Read the model definition and answer for the solid it produces. Units are mm, in the model's axes. A direction names the side the tool comes from. Coordinates: 2 decimals unless noted, no trailing zeros. Loops run counter-clockwise (first coordinate to the right, second up) from the corner with the lowest first, then second, coordinate; pieces in that order, holes last. Notation, with made-up numbers: (-25.75, 38) -> (0.25, 38) arc R17 cw to (0.25, 66) -> close; hole circle Ø1 at (41.25, -32). An arc over 180 degrees is marked (long way). Answer in a Markdown table with one row per item.
```python
from build123d import *

# Parameters (mm, degrees)
SKETCH1_W           = 109.5
SKETCH1_H           = 60.5
BOSS_EXTRUDE1_DEPTH = 14
SKETCH2_W           = 103.5
SKETCH2_H           = 54.5
CUT_EXTRUDE1_DEPTH  = 12
SKETCH4_W           = 13
SKETCH4_H           = 9
SKETCH4_W_2         = 10.2
CUT_EXTRUDE2_DEPTH  = 115.460964962
SKETCH5_W           = 4.5
SKETCH5_H           = 100
BOSS_EXTRUDE3_DEPTH = 4.8
BOSS_EXTRUDE7_DEPTH = 14
SKETCH9_W           = 50
SKETCH9_H           = 37.5
BOSS_EXTRUDE8_DEPTH = 4


with BuildPart() as part:
    # Sketch1 → Boss-Extrude1 (new body)
    with BuildSketch(Plane(origin=(0, 0, 0), x_dir=(1, 0, 0), z_dir=(0, 1, 0))):
        Rectangle(SKETCH1_W, SKETCH1_H)
    extrude(amount=BOSS_EXTRUDE1_DEPTH)

    # Sketch2 → Cut-Extrude1 (cut)
    with BuildSketch(Plane(origin=(0, 14, 0), x_dir=(1, 0, 0), z_dir=(0, 1, 0))):
        Rectangle(SKETCH2_W, SKETCH2_H)
    extrude(amount=-CUT_EXTRUDE1_DEPTH, mode=Mode.SUBTRACT)

    # Sketch4 → Cut-Extrude2 (cut, through all)
    with BuildSketch(Plane(origin=(54.75, 0, 0), x_dir=(0, 0, -1), z_dir=(1, 0, 0))):
        with Locations((-11.55, 9.5)):
            Rectangle(SKETCH4_W, SKETCH4_H)
        with Locations((18.25, 9.5)):
            Rectangle(SKETCH4_W_2, SKETCH4_H)
    extrude(amount=-CUT_EXTRUDE2_DEPTH, mode=Mode.SUBTRACT)

    # Sketch5 → Boss-Extrude3 (add)
    with BuildSketch(Plane.XZ):
        with Locations((-6.65, 19.75)):
            Rectangle(SKETCH5_W, SKETCH5_H)
    boss_extrude3 = extrude(amount=BOSS_EXTRUDE3_DEPTH)

    # Mirror1: Boss-Extrude3 across plane
    add(boss_extrude3.mirror(Plane(origin=(0, 0, 0), x_dir=(0, 0, 1), z_dir=(1, 0, 0))))

    # Sketch6 → Boss-Extrude7 (add)
    with BuildSketch(Plane(origin=(0, 0, 0), x_dir=(1, 0, 0), z_dir=(0, 1, 0))):
        Polygon((-0.75, -30.25), (-0.75, -69.75), (-54.75, -69.75), (-54.75, -30.25), (-52.75, -30.25), (-52.75, -67.75), (-2.75, -67.75), (-2.75, -30.25), align=None)
        Polygon((54.75, -30.25), (54.75, -69.75), (0.75, -69.75), (0.75, -30.25), (2.75, -30.25), (2.75, -67.75), (52.75, -67.75), (52.75, -30.25), align=None)
    extrude(amount=BOSS_EXTRUDE7_DEPTH)

    # Sketch9 → Boss-Extrude8 (add)
    with BuildSketch(Plane(origin=(0, 0, 0), x_dir=(1, 0, 0), z_dir=(0, 1, 0))):
        with Locations((-27.75, -49)):
            Rectangle(SKETCH9_W, SKETCH9_H)
        with Locations((27.75, -49)):
            Rectangle(SKETCH9_W, SKETCH9_H)
    extrude(amount=BOSS_EXTRUDE8_DEPTH)


solid = part.part
```
1. A cutting plane is placed at A-A on y = -3.25. Give the vertices of the cut face in (x, z).
A:
| item | result |
|---|---|
| outline | (-8.9, -30.25) -> (-4.4, -30.25) -> (-4.4, 69.75) -> (-8.9, 69.75) -> close; (4.4, -30.25) -> (8.9, -30.25) -> (8.9, 69.75) -> (4.4, 69.75) -> close |
2. A tool of negligible diameter and unlimited length cuts with its end or side. For faces 1 (the flat face through (53, 5, -18)), 2 (the flat face through (-53, 14, -4)), 3 (the flat face through (32, 0, 19)), 4 (the flat face through (51.75, 8, 0)), from which of +Z, -Z, +X, -X, +Y, -Y can it reach the whole face along a straight path? Write none if from no direction.
A:
| item | result |
|---|---|
| face 1 | +X, -X, +Y |
| face 2 | +Z, -Z, +X, -X, +Y |
| face 3 | +Z, -Z, +X, -Y |
| face 4 | +Y |
3. Find the intervals of material crossed by probe 1 along X at (y, z) = (10.25, 43); probe 2 along Z at (x, y) = (-27.5, 8); probe 3 along X at (y, z) = (-0.5, 52), in increasing order.
A:
| item | result |
|---|---|
| probe 1 | x = -54.75 to -52.75, -2.75 to -0.75, 0.75 to 2.75, 52.75 to 54.75 |
| probe 2 | z = -30.25 to -27.25, 27.25 to 30.25, 67.75 to 69.75 |
| probe 3 | x = -8.9 to -4.4, 4.4 to 8.9 |
4. A cutting plane is placed at C-C on y = 12.5. Count the separate pieces of the cut face and the enclosed holes in it, and give its area (3 significant figures).
A:
| item | result |
|---|---|
| separate pieces | 4 |
| enclosed holes | 2 |
| area | 1,360 mm2 |
5. Given pin 1 Ø1.5 at (x, z) = (53, -18) entering from +Y; pin 2 Ø8 at (x, y) = (-9.5, -1) entering from -Z; pin 3 Ø1.4 at (y, z) = (-1.5, 11.5) entering from -X; pin 4 Ø10 at (x, z) = (32, -3) entering from +Y, each flat-ended and moving along its own axis, determine where each tip first touches the part or whether it passes through.
A:
| item | result |
|---|---|
| pin 1 | stops at y = 5 |
| pin 2 | stops at z = -30.25 |
| pin 3 | stops at x = -8.9 |
| pin 4 | stops at y = 2 |
6. The mould has two halves that part along Z. Classify faces 5 (the flat face through (-28, 9, 67.75)), 6 (the flat face through (-4.4, -2, 19)), 7 (the flat face through (-2.75, 9, 49)), 8 (the flat face through (-27, 7, 69.75)): pulls with the +Z half, pulls with the -Z half, needs draft (parallel to the pull), parting line crosses it, or undercut.
A:
| item | result |
|---|---|
| face 5 | undercut |
| face 6 | needs draft |
| face 7 | undercut |
| face 8 | pulls with the +Z half |
7. A cutting plane is placed at B-B on z = 63. Give the vertices of the cut face in (x, y).
A:
| item | result |
|---|---|
| outline | (-54.75, 0) -> (-8.9, 0) -> (-8.9, -4.8) -> (-4.4, -4.8) -> (-4.4, 0) -> (-0.75, 0) -> (-0.75, 14) -> (-2.75, 14) -> (-2.75, 4) -> (-52.75, 4) -> (-52.75, 14) -> (-54.75, 14) -> close; (0.75, 0) -> (4.4, 0) -> (4.4, -4.8) -> (8.9, -4.8) -> (8.9, 0) -> (54.75, 0) -> (54.75, 14) -> (52.75, 14) -> (52.75, 4) -> (2.75, 4) -> (2.75, 14) -> (0.75, 14) -> close |
8. A cutting plane is placed at D-D on z = -11. Give the vertices of the cut face in (x, y).
A:
| item | result |
|---|---|
| outline | (-54.75, 0) -> (-8.9, 0) -> (-8.9, -4.8) -> (-4.4, -4.8) -> (-4.4, 0) -> (4.4, 0) -> (4.4, -4.8) -> (8.9, -4.8) -> (8.9, 0) -> (54.75, 0) -> (54.75, 14) -> (51.75, 14) -> (51.75, 2) -> (-51.75, 2) -> (-51.75, 14) -> (-54.75, 14) -> close |
